from build123d import *

# Parameters (mm, degrees)
F0_R     = 13.5
F0_R_2   = 10
F1_DEPTH = 1
F0_R_3   = 17.5
F2_DEPTH = 2
F0_R_4   = 20
F3_DEPTH = 7
F5_START = 4
F4_R     = 20
F4_R_2   = 16
F5_DEPTH = 3
F6_R     = 1
F7_R     = 10
F8_DEPTH = 1


with BuildPart() as f1:
    # F0 (on Top) → F1 (new body)
    with BuildSketch(Plane.XY):
        Circle(F0_R)
        Circle(F0_R_2, mode=Mode.SUBTRACT)
    extrude(amount=F1_DEPTH)

    # F0 (on Top) → F2 (join)
    with BuildSketch(Plane.XY):
        Circle(F0_R_3)
        Circle(F0_R, mode=Mode.SUBTRACT)
    extrude(amount=F2_DEPTH)

    # F0 (on Top) → F3 (join)
    with BuildSketch(Plane.XY):
        Circle(F0_R_4)
        Circle(F0_R_3, mode=Mode.SUBTRACT)
    extrude(amount=F3_DEPTH)

    # F4 (on Top) → F5 (join)
    with BuildSketch(Plane.XY.offset(F5_START)):
        Circle(F4_R)
        Circle(F4_R_2, mode=Mode.SUBTRACT)
    extrude(amount=F5_DEPTH)

    # F6
    f6_edges = [f1.edges().sort_by_distance(p)[0] for p in [
        (-16, 0, 4),
    ]]
    fillet(f6_edges, radius=F6_R)

    # F7 (on face) → F8 (join)
    with BuildSketch(Plane(origin=(0, 0, 0), x_dir=(1, 0, 0), z_dir=(0, 0, -1))):
        with BuildLine():
            add(Edge.make_bspline(
                [(0, 21.4875730586), (6.7657779426, 22.9365033035), (19.1072018799, 23.0482109616), (42.3023448655, 28.3031387355), (62.5173056226, 22.6182888102), (74.7384138035, 9.0261408273), (74.8955963135, 0)],
                knots=[0, 0, 0, 0, 0.2365573131, 0.4928095835, 0.735068508, 1, 1, 1, 1], degree=3))
            ThreePointArc((0, 21.4875730586), (-21.4875730586, 0), (0, -21.4875730586))
            add(Edge.make_bspline(
                [(0, -21.4875730586), (6.5654981556, -22.184182424), (20.8345654653, -25.1367847277), (37.794885628, -28.3962922072), (63.6423801672, -24.0427135063), (74.3739329381, -10.4370014279), (74.8955963135, 0)],
                knots=[0, 0, 0, 0, 0.2436300342, 0.4682692375, 0.7315377861, 1, 1, 1, 1], degree=3))
        make_face()
        Circle(F7_R, mode=Mode.SUBTRACT)
    extrude(amount=F8_DEPTH)


solid = f1.part
Verification items for the finished model (mm, model axes). A direction names the side the tool comes from. Give positions to 0.01 mm unless a question says otherwise; leave off trailing zeros. Order: outer loops, then holes, each group sorted by start corner. A loop starts at its lowest first (then second) coordinate and runs counter-clockwise, first axis right, second up. Notation, with made-up numbers: (80, -4.5) -> (122, -4.5) arc R17 ccw to (122, 15.5) -> close; hole circle Ø2 at (-31.5, -26.5). An arc over 180 degrees is marked (long way). Answer as CSV lines item,"result".
Q1. Scan lines: probe 1 along Y at (x, z) = (0, 6.5); probe 2 along Z at (x, y) = (13, -8); probe 3 along Y at (x, z) = (0, 0.3). Record each from-to range of solid material in increasing order.
Solutions:
probe 1,"y = -20 to -16, 16 to 20"
probe 2,"z = -1 to 2"
probe 3,"y = -20 to -10, 10 to 20"
Q2. Depth check by flat-ended pin: pin 1 (1.5 mm diameter, centred on x = 1, y = -8, fed in from -Z) (1 decimal); pin 2 (2 mm diameter, centred on y = 14, z = 4, fed in from -X); pin 3 (13.5 mm diameter, centred on x = 4.5, y = 3.5, fed in from +Z); pin 4 (16 mm diameter, centred on x = 8, y = -4.5, fed in from +Z). Enter the tip coordinate at first touch or a pass-through.
Solutions:
pin 1,"passes through"
pin 2,"stops at x = -15.2"
pin 3,"stops at z = 1"
pin 4,"stops at z = 7"
Q3. Release check for a two-part mould opening along Y. For faces 4 (the flat face through (-8.98, 13.43, 7)), 5 (the cylindrical face through (-2.17, 9.76, 0.01)), 6 (the cylindrical face through (-4.336, -19.524, 3.451)) record: +Y half, -Y half, draft (parallel to the pull), parting line (faces both ways), or undercut.
Solutions:
face 4,"draft"
face 5,"undercut"
face 6,"parting line"
Q4. Access from +Z, -Z, +X, -X, +Y, -Y to the whole of each face (thin tool, end or side, straight path). Record for faces 1 (the flat face through (27, 0, -1)), 2 (the flat face through (-3, 17, 4)), 3 (the cylindrical face through (-3.47, -15.62, 5.99)).
Solutions:
face 1,"-Z, +X, -X, +Y, -Y"
face 2,"none"
face 3,"+Z"
Q5. Sectioned sample at A-A on z = 3. Record the cut outline in (x, y), plus the area to 3 significant figures.
Solutions:
outline,"circle Ø40 at (0, 0); hole circle Ø35 at (0, 0)"
area,"295 mm²"
